The listing builds one solid part. Answer for the finished solid, in the listing's coordinates (mm). Face numbers are marked on the shaded views. Give positions to 0.01 mm unless a question says otherwise; leave off trailing zeros. Write each loop counter-clockwise with the first axis right and the second up, starting at its lowest first coordinate (ties: lowest second). Pieces come first, ordered by that corner, then holes. Notation, with made-up numbers: (28.5, 21.25) - (78.5, 21.25) arc R23 ccw to (78.5, 40.25) - close; hole circle Ø1 at (73, 52.25). An arc over 180 degrees is marked (long way). Use a Markdown table: item, result. Add a question column.
Autodesk Inventor part; units mm, degrees
ref_plane "YZ Plane" through (0, 0, 0) normal (1, 0, 0) x (0, 1, 0)
ref_plane "XZ Plane" through (0, 0, 0) normal (0, 1, 0) x (-1, 0, 0)
ref_plane "XY Plane" through (0, 0, 0) normal (0, 0, 1) x (1, 0, 0)
sketch "Sketch1" plane through (0, 0, 0) normal (0, 1, 0) x (-1, 0, 0)
  arc A0 (-40.2823, -25.1712) -> (38.9097, -27.2449) centre (0, 0) ccw
  line L0 (-40.2823, -25.1712) -> (-48.7628, -30.4704)
  line L1 (38.9097, -27.2449) -> (47.1012, -32.9806)
  arc A1 (-48.7628, -30.4704) -> (47.1012, -32.9806) centre (0, 0) ccw
  line L2 (0, -70.4825) -> (0, 11.7471) construction
  dimension "d0" = 47.5
  dimension "d1" = 57.5
  dimension "d2" = 55
  dimension "d3" = 58
extrude "Extrusion1" add sketch "Sketch1" along normal blind 5
sketch "Sketch2" plane through (0, 5, 0) normal (0, 1, 0) x (1, 0, 0)
  line L0 (40.2823, 25.1712) -> (48.7628, 30.4704)
  arc A0 (40.2823, 25.1712) -> (-38.9097, 27.2449) centre (0, 0) ccw
  arc A1 (48.7628, 30.4704) -> (-47.1012, 32.9806) centre (0, 0) ccw
  line L1 (22.2999, 41.94) -> (26.9946, 50.7695)
  dimension "d6" = 30
extrude "Extrusion2" add sketch "Sketch2" along normal blind 12
sketch "Sketch3" plane through (0, 17, 0) normal (0, 1, 0) x (1, 0, 0)
  circle A0 centre (41.9284, 31.5953) radius 1.5
  arc A1 (40.2823, 25.1712) -> (22.2999, 41.94) centre (0, 0) ccw construction
  arc A2 (48.7628, 30.4704) -> (26.9946, 50.7695) centre (0, 0) ccw construction
  line L0 (40.2823, 25.1712) -> (48.7628, 30.4704) construction
  line L1 (26.9946, 50.7695) -> (22.2999, 41.94) construction
  line L2 (37.9352, 28.5862) -> (45.9215, 34.6044) construction
  line L3 (32.3949, 34.7393) -> (39.2149, 42.0528) construction
  circle A3 centre (35.8049, 38.3961) radius 1.5
  dimension "d9" = 3
  dimension "d10" = 5
  dimension "d11" = 15
extrude "Extrusion3" cut sketch "Sketch3" against normal up to surface (17 mm away)
properties part number "Right_Bottom_Gripper"
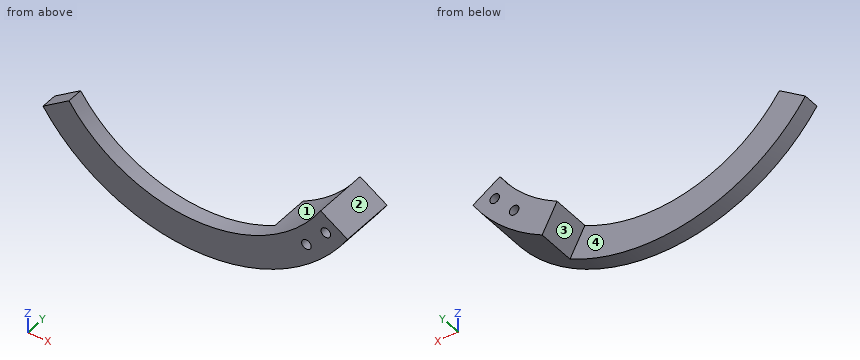
1. The part is cut by section C-C (z = -44). Give the vertices of the cut face in (x, y), and give its area (3 significant figures).
2. For a pull along X with two mould halves and no side action, classify the marked faces 1, 2, 3 and 4 as released by +X, released by -X, zero draft, split by the parting line, or undercut.
3. The part is cut by section D-D (x = -26). Give the vertices of the cut face in (y, z).
4. The part is cut by section A-A (z = -29). Give the vertices of the cut face in (x, y).
5. Given P1, Ø1.8, axis at x = 41.93, z = -31.6, coming from the +Y side; P2, Ø5, axis at y = 5, z = -48.5, coming from the +X side; P3, Ø6, axis at y = 3, z = -36, coming from the +X side; P4, Ø6, axis at x = -6, z = -48.5, coming from the +Y side, each flat-ended and moving along its own axis, determine where each tip first touches the part or whether it passes through.
6. Consider L1, parallel to Y at x = -35.5, z = -38.5; L2, parallel to X at y = 10, z = -31; L3, parallel to Z at x = 35, y = 6. Determine where each line is inside the solid, lowest interval first. Write a range as [from, to].
7. The part is cut by section B-B (y = 8). Give the vertices of the cut face in (x, z).
Check values:
| question | item | result |
|---|---|---|
| 1 | outline | (-37.02, 0) - (-17.9, 0) - (-17.9, 5) - (-37.02, 5) - close; (17.9, 0) - (37.02, 0) - (37.02, 17) - (23.4, 17) - (23.4, 5) - (17.9, 5) - close |
| 1 | area | 355 mm2 |
| 2 | face 1 | undercut |
| 2 | face 2 | released by +X |
| 2 | face 3 | released by -X |
| 2 | face 4 | zero draft |
| 3 | outline | (0, -51.29) - (5, -51.29) - (5, -39.75) - (0, -39.75) - close |
| 4 | outline | (-41.42, 0) - (-37.62, 0) - (-37.62, 5) - (-41.42, 5) - close; (37.62, 0) - (46.41, 0) - (46.41, 17) - (37.62, 17) - close |
| 5 | P1 | passes through |
| 5 | P2 | stops at x = 34.5 |
| 5 | P3 | stops at x = 47.09 |
| 5 | P4 | stops at y = 5 |
| 6 | L1 | y = [0, 5] |
| 6 | L2 | x = [35.99, 40.55], [43.31, 48.43] |
| 6 | L3 | z = [-45.62, -39.66], [-37.13, -32.11] |
| 7 | outline | (22.3, -41.94) - (26.99, -50.77) arc R57.5 ccw to (48.76, -30.47) - (40.28, -25.17) arc R47.5 cw to start; hole circle Ø3 at (35.8, -38.4); hole circle Ø3 at (41.93, -31.6) |
